Here's how the part is built. I have some questions about the finished solid (model axes, mm). A direction names the side the tool comes from. Round coordinates to 2 decimals unless told otherwise and drop trailing zeros. Write each loop counter-clockwise with the first axis right and the second up, starting at its lowest first coordinate (ties: lowest second). Pieces come first, ordered by that corner, then holes. Notation, with made-up numbers: (74, 23.5) - (88, 23.5) arc R21 cw to (88, 33.5) - close; hole circle Ø2 at (-7, -2.75). An arc over 180 degrees is marked (long way). Use one line per item in the form item = value. Start each with the question number.
1. If I drill on line 1 along X through (y, z) = (-20, -25); line 2 along Z through (x, y) = (0, -9.5); line 3 along Z through (x, y) = (60.5, -18.75), over which ranges is the centre line in solid material (lowest first)?
2. Will this pin go through, and if not, where does the flat tip stop? pin 1 (18 mm diameter, centred on x = 0, z = -25, fed in from -Y).
3. I want a section at B-B, the plane z = -25. List the corners of the cut face in (x, y) for me.
4. I want a section at A-A, the plane x = 0. List the corners of the cut face in (y, z) for me, plus the area to 3 significant figures.
5. I want a section at C-C, the plane y = -16.5. List the corners of the cut face in (x, z) for me, plus the area to 3 significant figures.
6. We'd pull the mould along X, two halves only. Please class faces 3 (the flat face through (100, -12, -25)), 4 (the flat face through (-1, -12, -50)), 5 (the cylindrical face through (39, -12, -25)): +X half, -X half, draft (parallel to the pull), parting line (faces both ways), or undercut.
7. I want a section at D-D, the plane x = 48. List the corners of the cut face in (y, z) for me, plus the area to 3 significant figures.
8. Which directions (+Z, -Z, +X, -X, +Y, -Y) give clear straight access to the entire face, cutting with the end or side of a thin tool? Please do faces 1 (the flat face through (-100, -12, -25)), 2 (the cylindrical face through (-39, -12, -25)).
```python
from build123d import *

# Parameters (mm, degrees)
F0_W     = 200
F0_H     = 50
F1_DEPTH = 25
F2_D     = 14


with BuildPart() as f1:
    # F0 (on Front) → F1 (new body)
    with BuildSketch(Plane.XZ):
        with Locations((0, -25)):
            Rectangle(F0_W, F0_H)
        with BuildLine():
            Line((-55, -41), (-65, -41))
            ThreePointArc((-65, -41), (-81, -25), (-65, -9))
            Line((-65, -9), (-55, -9))
            ThreePointArc((-55, -9), (-39, -25), (-55, -41))
        make_face(mode=Mode.SUBTRACT)
        with BuildLine():
            Line((55, -9), (65, -9))
            ThreePointArc((65, -9), (81, -25), (65, -41))
            Line((65, -41), (55, -41))
            ThreePointArc((55, -41), (39, -25), (55, -9))
        make_face(mode=Mode.SUBTRACT)
    extrude(amount=F1_DEPTH)

    # F2 (through all)
    with Locations(Plane(origin=(0, 0, 0), x_dir=(1, 0, 0), z_dir=(0, 1, 0))):
        with Locations((0, 25)):
            Hole(F2_D / 2)


solid = f1.part
```
Model answer:
q1.line_1 = -100 to -81, -39 to -7, 7 to 39, 81 to 100
q1.line_2 = -50 to -32, -18 to 0
q1.line_3 = -50 to -41, -9 to 0
q2.pin_1 = -25
q3.outline = (-100, -25) - (-81, -25) - (-81, 0) - (-100, 0) - close; (-39, -25) - (-7, -25) - (-7, 0) - (-39, 0) - close; (7, -25) - (39, -25) - (39, 0) - (7, 0) - close; (81, -25) - (100, -25) - (100, 0) - (81, 0) - close
q4.outline = (-25, -50) - (0, -50) - (0, -32) - (-25, -32) - close; (-25, -18) - (0, -18) - (0, 0) - (-25, 0) - close
q4.area = 900 mm2
q5.outline = (-100, -50) - (100, -50) - (100, 0) - (-100, 0) - close; hole (-65, -41) - (-55, -41) arc R16 ccw to (-55, -9) - (-65, -9) arc R16 ccw to start; hole circle Ø14 at (0, -25); hole (55, -41) - (65, -41) arc R16 ccw to (65, -9) - (55, -9) arc R16 ccw to start
q5.area = 7,600 mm2
q6.face_3 = +X half
q6.face_4 = draft
q6.face_5 = undercut
q7.outline = (-25, -50) - (0, -50) - (0, -39.39) - (-25, -39.39) - close; (-25, -10.61) - (0, -10.61) - (0, 0) - (-25, 0) - close
q7.area = 531 mm2
q8.face_1 = +Z, -Z, -X, +Y, -Y
q8.face_2 = +Y, -Y
